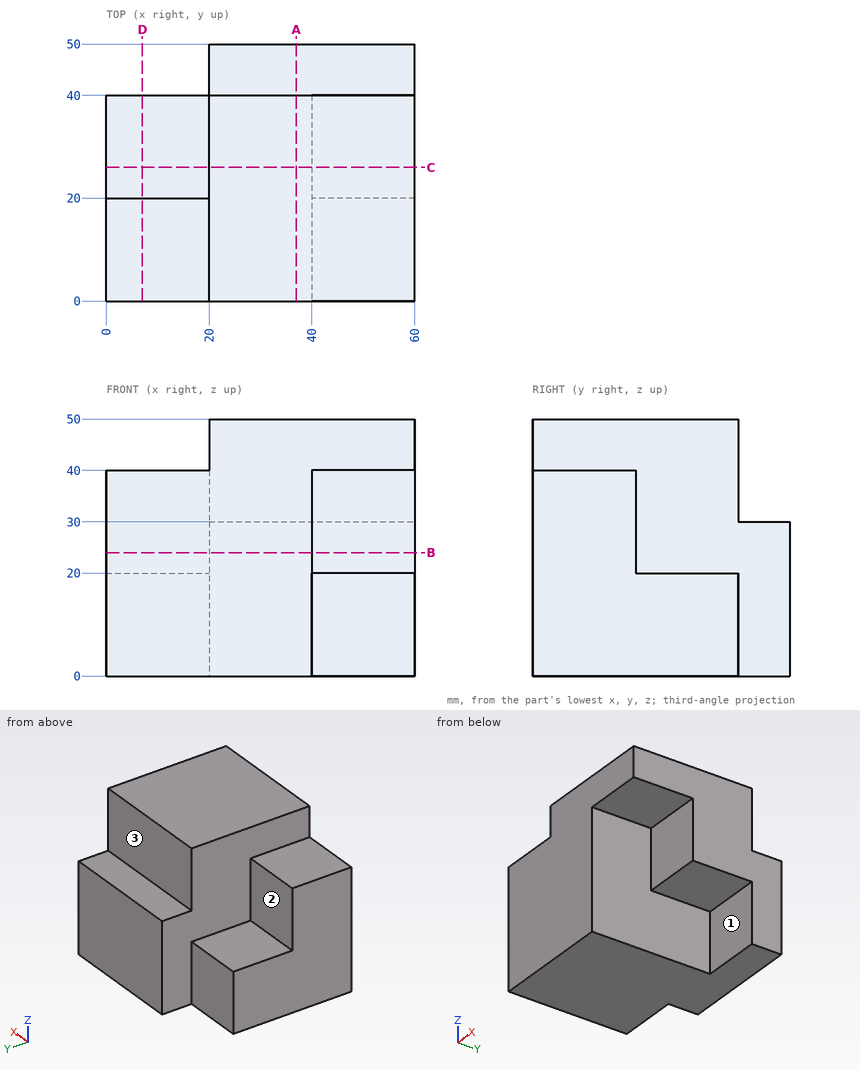
The drawing under review shows one solid part. Ordinate dimensions are in mm from its lowest x, y, z. A direction names the side the tool comes from. Coordinates: 2 decimals unless noted, no trailing zeros. Order: outer loops, then holes, each group sorted by start corner. A loop starts at its lowest first (then second) coordinate and runs counter-clockwise, first axis right, second up. Notation, with made-up numbers: (-0.75, 48) - (52.25, 48) arc R21 cw to (52.25, 53) - close; hole circle Ø3 at (12, -10). An arc over 180 degrees is marked (long way). Put each result on its own line as item: value.
1) Tool access review of the marked faces 1, 2 and 3: name each direction out of +Z, -Z, +X, -X, +Y, -Y from which nothing blocks a thin tool from reaching the whole face with its end or side.
Response values:
face 1: -Z, +X, -Y
face 2: +Z, -X, +Y
face 3: +Z, +X, -X, +Y
2) Wall thickness on L1, parallel to Y at x = 23, z = 42.5; L2, parallel to X at y = 29, z = 33.5: over which ranges is each line inside the solid? List them lowest first. Write a range as from..to.
Response values:
L1: y = 0..40
L2: x = 20..60
3) Take a section at B-B, the plane z = 24. Give the boundary of the cut face in (x, y), and give its area (3 significant figures).
Response values:
outline: (0, 0) - (40, 0) - (40, 20) - (60, 20) - (60, 50) - (20, 50) - (20, 20) - (0, 20) - close
area: 2,000 mm²
4) Take a section at A-A, the plane x = 37. Give the boundary of the cut face in (y, z).
Response values:
outline: (0, 0) - (50, 0) - (50, 30) - (40, 30) - (40, 50) - (0, 50) - close
5) Take a section at D-D, the plane x = 7. Give the boundary of the cut face in (y, z), and give its area (3 significant figures).
Response values:
outline: (0, 0) - (40, 0) - (40, 20) - (20, 20) - (20, 40) - (0, 40) - close
area: 1,200 mm²
6) Insertion check: P1, Ø6, axis at x = 11, y = 8.5, coming from the +Z side; P2, Ø5, axis at y = 19.5, z = 12, coming from the +X side; P3, Ø5, axis at x = 46.5, y = 43, coming from the +Z side. Each pin has a flat end and moves straight along its axis. Give the tip position at first contact, or say it passes through.
Response values:
P1: stops at z = 40
P2: stops at x = 40
P3: stops at z = 30
